```python
from build123d import *

# Parameters (mm, degrees)
F0_R      = 69.85
F1_DEPTH  = 571.5
F2_R      = 65.405
F3_DEPTH  = 146.0754
F3_FACE_R = 65.405
F5_R      = 41.275
F7_R      = 41.275
F8_DEPTH  = 50.8
F10_D     = 19.05
F10_DEPTH = 53.975
F10_TIP   = 5.7231973962


with BuildPart() as f1:
    # F0 (on Right) → F1 (new body, symmetric)
    with BuildSketch(Plane.YZ):
        Circle(F0_R)
    extrude(amount=F1_DEPTH, both=True)

    # F2 (on face) → F3 (join)
    with BuildSketch(Plane.YZ.offset(571.5)):
        Circle(F2_R)
    extrude(amount=F3_DEPTH)

    # F3_face (on face) → F6 section 0
    with BuildSketch(Plane.YZ.offset(717.5754)):
        Circle(F3_FACE_R)
    # F5 (on offset) → F6 section 1
    with BuildSketch(Plane.YZ.offset(863.6254)):
        Circle(F5_R)
    loft()

    # F7 (on face) → F8 (join)
    with BuildSketch(Plane.YZ.offset(863.6254)):
        Circle(F7_R)
    extrude(amount=F8_DEPTH)

    # F10
    with Locations(Plane.YZ.offset(914.4254)):
        with Locations((0, 0)):
            Hole(F10_D / 2, depth=F10_DEPTH)
            with Locations((0, 0, -(F10_DEPTH + F10_TIP / 2))):  # 118° drill point
                Cone(0, F10_D / 2, F10_TIP, mode=Mode.SUBTRACT)

    # F11: F1 across plane


with BuildPart() as f1_1:
    add(f1.part)
    add(f1.part.mirror(Plane.YZ))


solid = f1_1.part
```
Model file for the job. Use its own axes, mm. A direction names the side the tool comes from. Give positions to 0.01 mm unless a question says otherwise; leave off trailing zeros. Write each loop counter-clockwise with the first axis right and the second up, starting at its lowest first coordinate (ties: lowest second). Pieces come first, ordered by that corner, then holes. Notation, with made-up numbers: (69, 57.5) - (79, 57.5) arc R12 ccw to (79, 70.5) - close; hole circle Ø10 at (17, -6.75). An arc over 180 degrees is marked (long way). One line per question, with ' | ' between items. Start each with the question number.
(1) Slice it at A-A on x = -605. Write the cut outline in (y, z) (3 decimals), plus the area to 3 significant figures.
(2) 3-axis set-ups, long thin cutter, end or side, ignore diameter. For faces 1 (the face through (-571.5, 20.4, 62.4)), 2 (the face through (-914.425, -1, 10)), 3 (the face through (571.5, 20.4, 62.4)): which of +Z, -Z, +X, -X, +Y, -Y reach the whole face in a straight line?
(3) Pin check, flat tips, straight feed: P1, Ø5, axis at x = -458, y = 34, coming from the -Z side; P2, Ø1, axis at y = 48, z = 47.5, coming from the +X side; P3, Ø1, axis at x = 219.5, z = 21, coming from the -Y side. Stop position of each tip, or through.
(4) Wall check: line 1 along Z through (x, y) = (-895, 0) (3 decimals); line 2 along Y through (x, z) = (-741.5, 45.5); line 3 along X through (y, z) = (-57.5, 39.5). Give the ranges that are in metal, low to high. Write a range as from..to.
Results below:
1) outline: circle Ø130.81 at (0, 0) | area: 13,400 mm^2
2) face 1: -X | face 2: +Z, -Z, -X, +Y, -Y | face 3: +X
3) P1: z = -62.34 | P2: x = 571.5 | P3: y = -66.77
4) line 1: -41.275..-9.525, 9.525..41.275 | line 2: -41.31..41.31 | line 3: -571.5..571.5
